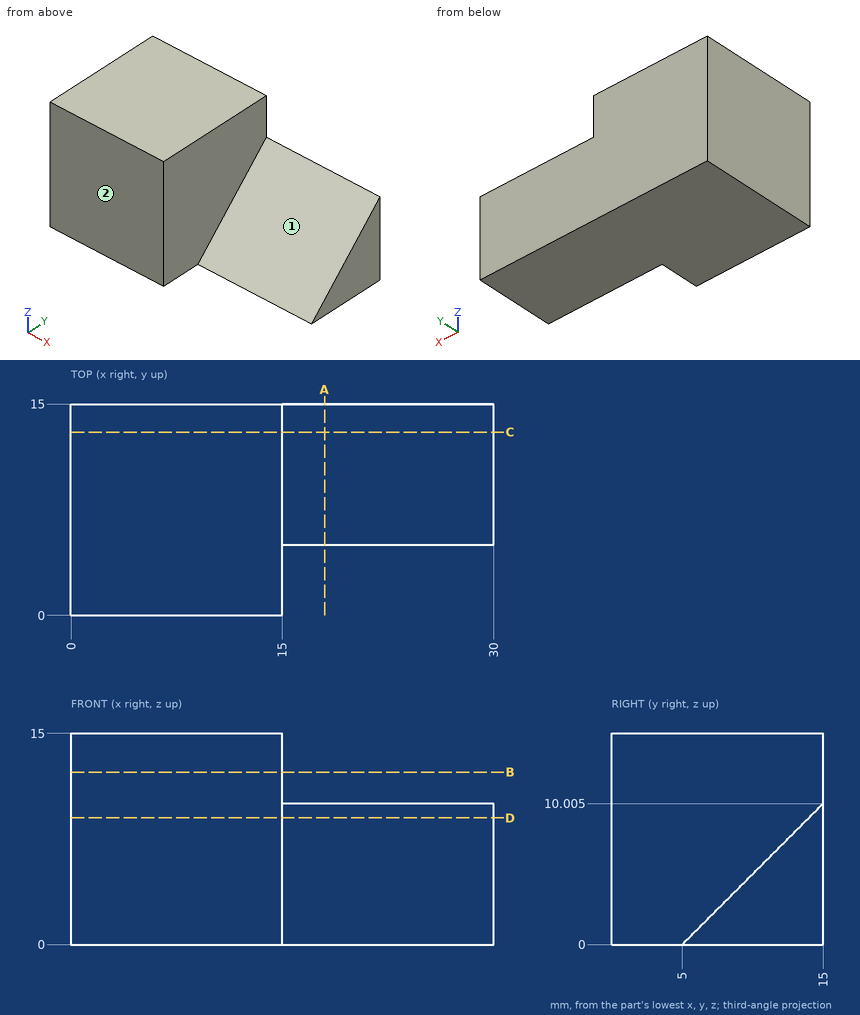
The figure shows three views and two pictorial views of one solid part (mm, origin at its lowest corner). Answer the questions. A direction names the side the tool comes from. Give positions to 0.01 mm unless a question says otherwise; leave off trailing zeros. Loops run counter-clockwise (first coordinate to the right, second up) from the corner with the lowest first, then second, coordinate; pieces in that order, holes last. Notation, with made-up numbers: (-26, 45.5) -> (24, 45.5) arc R25 ccw to (24, 59.5) -> close; hole circle Ø1 at (-4.5, 81). An arc over 180 degrees is marked (long way). Use CSV: the item, a comma, the result in double quotes.
1. The part is cut by section D-D (z = 9). Write down the section's boundary in (x, y).
Found:
outline,"(0, 0) -> (15, 0) -> (15, 14) -> (30, 14) -> (30, 15) -> (0, 15) -> close"
2. The part is cut by section B-B (z = 12.25). Write down the section's boundary in (x, y), then the cut area to 3 significant figures.
Found:
outline,"(0, 0) -> (15, 0) -> (15, 15) -> (0, 15) -> close"
area,"225 mm^2"
3. A tool of negligible diameter and unlimited length cuts with its end or side. For the marked faces 1 and 2, from which of +Z, -Z, +X, -X, +Y, -Y can it reach the whole face along a straight path? Write none if from no direction.
Found:
face 1,"+Z, +X, -Y"
face 2,"+Z, -Z, +X, -X, -Y"
4. The part is cut by section A-A (x = 18). Write down the section's boundary in (y, z) (3 decimals), then the cut area to 3 significant figures.
Found:
outline,"(5, 0) -> (15, 0) -> (15, 10.005) -> close"
area,"50.0 mm^2"
5. The part is cut by section C-C (y = 13). Write down the section's boundary in (x, z), then the cut area to 3 significant figures.
Found:
outline,"(0, 0) -> (30, 0) -> (30, 8) -> (15, 8) -> (15, 15) -> (0, 15) -> close"
area,"345 mm^2"
6. Flat-ended cylindrical pins translate along their axes: pin 1 Ø5 at (y, z) = (3.5, 4) entering from +X; pin 2 Ø4 at (x, z) = (20, 4.5) entering from -Y. Find the tip coordinate at first contact, or state that the pin passes through.
Found:
pin 1,"x = 15"
pin 2,"y = 7.5"
7. Straight lines are drawn through the part: line 1 (X direction, y = 6.25, z = 10); line 2 (Z direction, x = 24.5, y = 14.5) (1 decimal); line 3 (Y direction, x = 16.25, z = 3). For each, find the intervals that lie inside material, in ascending order.
Found:
line 1,"0 to 15"
line 2,"0 to 9.5"
line 3,"8 to 15"
